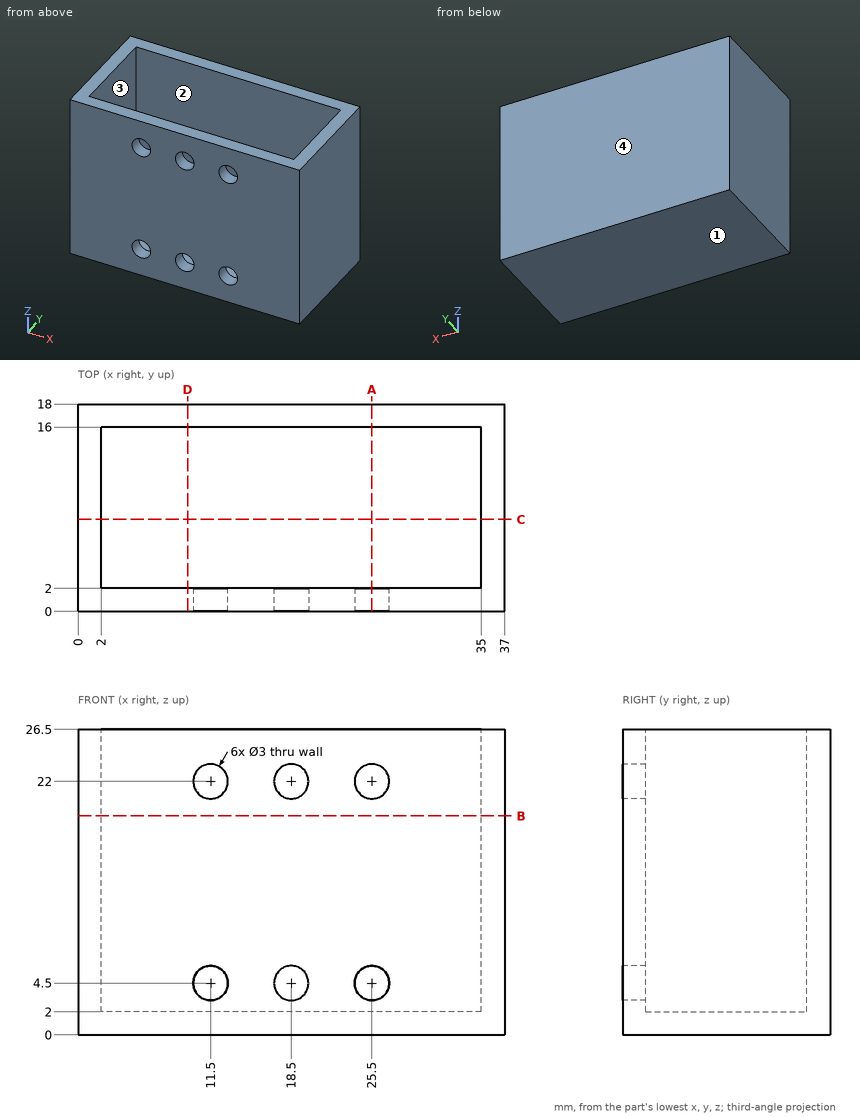
Geometry: see drawing. Coordinates: mm, zero at the bounding-box minimum. Coordinates: 2 decimals unless noted, no trailing zeros. Order: outer loops, then holes, each group sorted by start corner. A loop starts at its lowest first (then second) coordinate and runs counter-clockwise, first axis right, second up. Notation, with made-up numbers: M -24.75,57 L -12.75,57 A21 ccw -12.75,72 Z; hole C 75.5,46 d10. An arc over 180 degrees is marked long. Write item = value, one per line. Start each with the question number.
(1) Pull-direction query (Y, two-part tool) for the marked faces 1, 2, 3 and 4; classes: released by +Y, released by -Y, zero draft, split by the parting line, or undercut.
(2) Section D-D on x = 9.5. Output: boundary loops of the cut face in (y, z).
(3) Section A-A on x = 25.5. Output: boundary loops of the cut face in (y, z), and give its area (3 significant figures).
(4) Line query: line 1 along Z through (x, y) = (25.5, 0.8); line 2 along Y through (x, z) = (6, 12.25); line 3 along X through (y, z) = (8, 17). Output: solid intervals per line, ascending. Write a range as [from, to].
(5) Section B-B on z = 19. Output: boundary loops of the cut face in (x, y).
(6) First-contact query: P1, Ø7, axis at x = 12, y = 8.5, coming from the +Z side; P2, Ø1.8, axis at x = 11.5, z = 22, coming from the -Y side. Flat tips, straight axial feed; report the tip coordinate or a pass-through.
(7) Section C-C on y = 8. Output: boundary loops of the cut face in (x, z).
Result set:
q1.face_1 = zero draft
q1.face_2 = undercut
q1.face_3 = undercut
q1.face_4 = released by +Y
q2.outline = M 0,0 L 18,0 L 18,26.5 L 16,26.5 L 16,2 L 2,2 L 2,26.5 L 0,26.5 Z
q3.outline = M 0,0 L 18,0 L 18,26.5 L 16,26.5 L 16,2 L 2,2 L 2,3 L 0,3 Z; M 0,6 L 2,6 L 2,20.5 L 0,20.5 Z; M 0,23.5 L 2,23.5 L 2,26.5 L 0,26.5 Z
q3.area = 122 mm²
q4.line_1 = [0, 3], [6, 20.5], [23.5, 26.5]
q4.line_2 = [0, 2], [16, 18]
q4.line_3 = [0, 2], [35, 37]
q5.outline = M 0,0 L 37,0 L 37,18 L 0,18 Z; hole M 2,2 L 35,2 L 35,16 L 2,16 Z
q6.P1 = 2
q6.P2 = 16
q7.outline = M 0,0 L 37,0 L 37,26.5 L 35,26.5 L 35,2 L 2,2 L 2,26.5 L 0,26.5 Z
